Part print with two shaded views. Sizes in mm from the minimum x, y, z corner. Round coordinates to 2 decimals unless told otherwise and drop trailing zeros. Write each loop counter-clockwise with the first axis right and the second up, starting at its lowest first coordinate (ties: lowest second). Pieces come first, ordered by that corner, then holes. Notation, with made-up numbers: (-23.75, 45) -> (4.25, 45) arc R23 cw to (4.25, 66) -> close; hole circle Ø2 at (69.5, 53). An arc over 180 degrees is marked (long way). Answer as CSV lines item,"result".
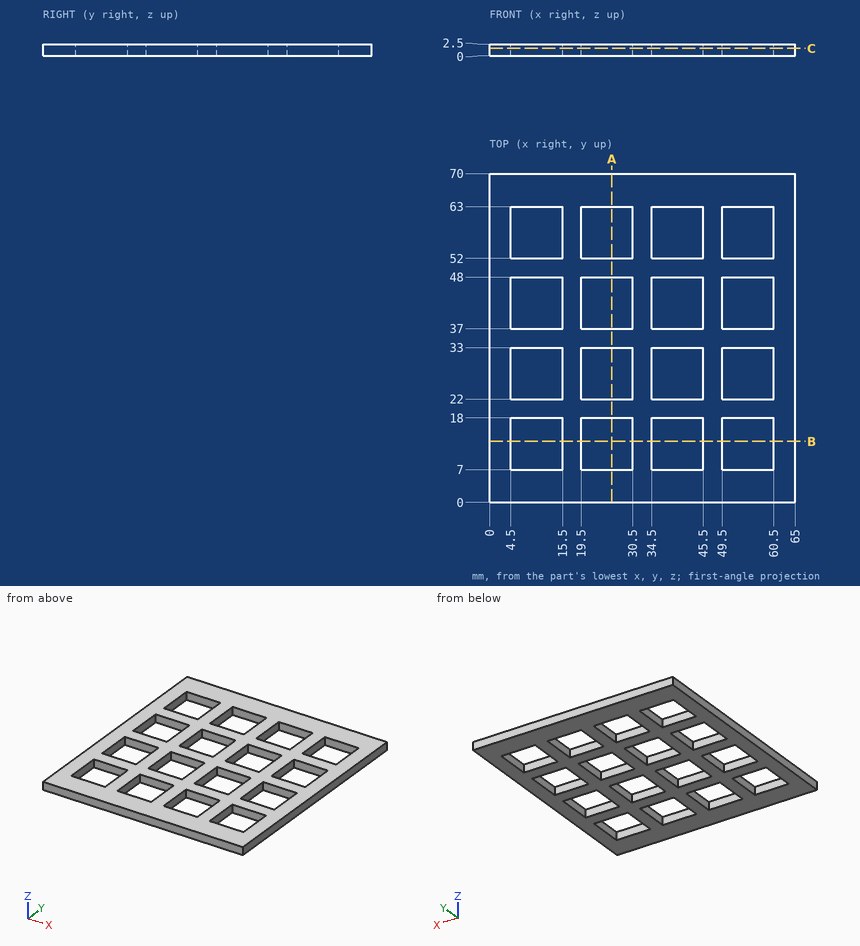
1. Cut at B-B, the plane y = 13. Write the cut outline in (x, z).
Results found:
outline,"(0, 0) -> (4.5, 0) -> (4.5, 2.5) -> (0, 2.5) -> close; (15.5, 0) -> (19.5, 0) -> (19.5, 2.5) -> (15.5, 2.5) -> close; (30.5, 0) -> (34.5, 0) -> (34.5, 2.5) -> (30.5, 2.5) -> close; (45.5, 0) -> (49.5, 0) -> (49.5, 2.5) -> (45.5, 2.5) -> close; (60.5, 0) -> (65, 0) -> (65, 2.5) -> (60.5, 2.5) -> close"
2. Probe line 1 along Y through (x, z) = (44, 0.2); line 2 along X through (y, z) = (17, 1.95). List the from-to ranges inside material, lowest first.
Results found:
line 1,"y = 0 to 7, 18 to 22, 33 to 37, 48 to 52, 63 to 70"
line 2,"x = 0 to 4.5, 15.5 to 19.5, 30.5 to 34.5, 45.5 to 49.5, 60.5 to 65"
3. Cut at A-A, the plane x = 26. Write the cut outline in (y, z).
Results found:
outline,"(0, 0) -> (7, 0) -> (7, 2.5) -> (0, 2.5) -> close; (18, 0) -> (22, 0) -> (22, 2.5) -> (18, 2.5) -> close; (33, 0) -> (37, 0) -> (37, 2.5) -> (33, 2.5) -> close; (48, 0) -> (52, 0) -> (52, 2.5) -> (48, 2.5) -> close; (63, 0) -> (70, 0) -> (70, 2.5) -> (63, 2.5) -> close"
4. Cut at C-C, the plane z = 1.55. Count the separate pieces of the cut face and the enclosed holes in it, then the cut area to 3 significant figures.
Results found:
separate pieces,"1"
enclosed holes,"16"
area,"2,610 mm2"
